The listing builds one solid part. Answer for the finished solid, in the listing's coordinates (mm). Face numbers are marked on the shaded views. A direction names the side the tool comes from. Coordinates: 2 decimals unless noted, no trailing zeros. Write each loop counter-clockwise with the first axis right and the second up, starting at its lowest first coordinate (ties: lowest second). Pieces come first, ordered by that corner, then holes.
```python
from build123d import *

# Parameters (mm, degrees)
SKETCH1_R                                    = 1.5
BOSS_EXTRUDE1_DEPTH                          = 1.2
BOSS_EXTRUDE1_2_DEPTH                        = 1.2
BOSS_EXTRUDE1_3_DEPTH                        = 1.2
SKETCH2_R                                    = 1.5
BOSS_EXTRUDE2_DEPTH                          = 3.5
SKETCH3_R                                    = 1.5
BOSS_EXTRUDE3_DEPTH                          = 1
CSK_FOR_M3_COUNTERSUNK_FLAT_HEAD_SCR_2_COUNT = 2
CSK_FOR_M3_COUNTERSUNK_FLAT_HEAD_SCR_2_PITCH = 19
CSK_FOR_M3_COUNTERSUNK_FLAT_HEAD_SCR_3_COUNT = 2
CSK_FOR_M3_COUNTERSUNK_FLAT_HEAD_SCR_3_PITCH = 38
SKETCH7_R                                    = 3
CUT_EXTRUDE1_DEPTH                           = 67.004185473
SKETCH8_W                                    = 6.5
SKETCH8_H                                    = 3.5
CUT_EXTRUDE2_DEPTH                           = 67.004185473
SKETCH10_W                                   = 9.5
SKETCH10_H                                   = 1.1
CUT_EXTRUDE3_DEPTH                           = 1


with BuildPart() as part:
    # Sketch1 → Boss-Extrude1 (new body)
    with BuildSketch(Plane.XY):
        Polygon((-55.55, 8.6), (-54.75, 8.6), (-54.75, 14), (-64.25, 14), (-64.25, 0), (-54.75, 0), (-54.75, 4.6), (-55.55, 4.6), align=None)
        with Locations((-59.5, 9.5)):
            Circle(SKETCH1_R, mode=Mode.SUBTRACT)
    extrude(amount=BOSS_EXTRUDE1_DEPTH)



with BuildPart() as body_2:
    # Sketch1 → Boss-Extrude1 2 (new body)
    with BuildSketch(Plane.XY):
        Polygon((-45.25, 4.6), (-45.25, 0), (-35.75, 0), (-35.75, 4.6), (-36.55, 4.6), (-36.55, 8.6), (-35.75, 8.6), (-35.75, 14), (-45.25, 14), (-45.25, 8.6), (-44.45, 8.6), (-44.45, 4.6), align=None)
        with Locations((-40.5, 9.5)):
            Circle(SKETCH1_R, mode=Mode.SUBTRACT)
    extrude(amount=BOSS_EXTRUDE1_2_DEPTH)


with BuildPart() as body_3:
    # Sketch1 → Boss-Extrude1 3 (new body)
    with BuildSketch(Plane.XY):
        Polygon((-26.25, 4.6), (-26.25, 0), (-16.75, 0), (-16.75, 14), (-26.25, 14), (-26.25, 8.6), (-25.45, 8.6), (-25.45, 4.6), align=None)
        with Locations((-21.5, 9.5)):
            Circle(SKETCH1_R, mode=Mode.SUBTRACT)
    extrude(amount=BOSS_EXTRUDE1_3_DEPTH)


with BuildPart() as part_1:
    add(part.part)

    add(body_2.part)  # Boss-Extrude2 merges body 2

    add(body_3.part)  # Boss-Extrude2 merges body 3
    # Sketch2 → Boss-Extrude2 (add)
    with BuildSketch(Plane.XY.offset(1.2)):
        Polygon((-54.75, 14), (-64.25, 14), (-64.25, 0), (-16.75, 0), (-16.75, 14), (-26.25, 14), (-26.25, 1.1), (-35.75, 1.1), (-35.75, 14), (-45.25, 14), (-45.25, 1.1), (-54.75, 1.1), align=None)
        with Locations((-59.5, 9.5)):
            Circle(SKETCH2_R, mode=Mode.SUBTRACT)
        with Locations((-40.5, 9.5)):
            Circle(SKETCH2_R, mode=Mode.SUBTRACT)
        with Locations((-21.5, 9.5)):
            Circle(SKETCH2_R, mode=Mode.SUBTRACT)
    extrude(amount=BOSS_EXTRUDE2_DEPTH)

    # Sketch3 → Boss-Extrude3 (add)
    with BuildSketch(Plane.XY.offset(4.7)):
        Polygon((-64.25, 14), (-54.75, 14), (-54.75, 12.1), (-45.25, 12.1), (-45.25, 14), (-35.75, 14), (-35.75, 12.1), (-26.25, 12.1), (-26.25, 14), (-16.75, 14), (-16.75, 0), (-64.25, 0), align=None)
        with Locations((-59.5, 9.5)):
            Circle(SKETCH3_R, mode=Mode.SUBTRACT)
        with Locations((-40.5, 9.5)):
            Circle(SKETCH3_R, mode=Mode.SUBTRACT)
        with Locations((-21.5, 9.5)):
            Circle(SKETCH3_R, mode=Mode.SUBTRACT)
    extrude(amount=BOSS_EXTRUDE3_DEPTH)

    # Sketch6 → CSK for M3 Countersunk Flat Head Screw1 (revolve, cut)
    with BuildSketch(Plane(origin=(-59.5, 9.5, 5.7), x_dir=(0, -1, 0), z_dir=(1, 0, 0))):
        Polygon((0, 0), (0, 5.7), (1.7, 5.7), (1.7, 1.75), (3.15, 0.3), (3.15, 0), align=None)
    csk_for_m3_countersunk_flat_head_screw1 = revolve(axis=Axis((-59.5, 9.5, 12.05), (0, 0, -1)), mode=Mode.SUBTRACT)

    # CSK for M3 Countersunk Flat Head Scr 2: CSK for M3 Countersunk Flat Head Screw1 ×2
    with Locations(*[(i * CSK_FOR_M3_COUNTERSUNK_FLAT_HEAD_SCR_2_PITCH, 0, 0) for i in range(1, CSK_FOR_M3_COUNTERSUNK_FLAT_HEAD_SCR_2_COUNT)]):
        add(csk_for_m3_countersunk_flat_head_screw1, mode=Mode.SUBTRACT)

    # CSK for M3 Countersunk Flat Head Scr 3: CSK for M3 Countersunk Flat Head Screw1 ×2
    with Locations(*[(i * CSK_FOR_M3_COUNTERSUNK_FLAT_HEAD_SCR_3_PITCH, 0, 0) for i in range(1, CSK_FOR_M3_COUNTERSUNK_FLAT_HEAD_SCR_3_COUNT)]):
        add(csk_for_m3_countersunk_flat_head_screw1, mode=Mode.SUBTRACT)

    # Sketch7 → Cut-Extrude1 (cut, through all)
    with BuildSketch(Plane.XY.offset(5.7)):
        with Locations((-50, 6)):
            Circle(SKETCH7_R)
        with Locations((-31, 6)):
            Circle(SKETCH7_R)
    extrude(amount=-CUT_EXTRUDE1_DEPTH, mode=Mode.SUBTRACT)

    # Sketch8 → Cut-Extrude2 (cut, through all)
    with BuildSketch(Plane.XY.offset(5.7)):
        with Locations((-61, 1.75)):
            Rectangle(SKETCH8_W, SKETCH8_H)
        with Locations((-20, 1.75)):
            Rectangle(SKETCH8_W, SKETCH8_H)
    extrude(amount=-CUT_EXTRUDE2_DEPTH, mode=Mode.SUBTRACT)

    # Sketch10 → Cut-Extrude3 (cut)
    with BuildSketch(Plane(origin=(0, 0, 1.2), x_dir=(-1, 0, 0), z_dir=(0, 0, -1))):
        with Locations((31, 0.55)):
            Rectangle(SKETCH10_W, SKETCH10_H)
        with Locations((50, 0.55)):
            Rectangle(SKETCH10_W, SKETCH10_H)
    extrude(amount=-CUT_EXTRUDE3_DEPTH, mode=Mode.SUBTRACT)


solid = part_1.part
```
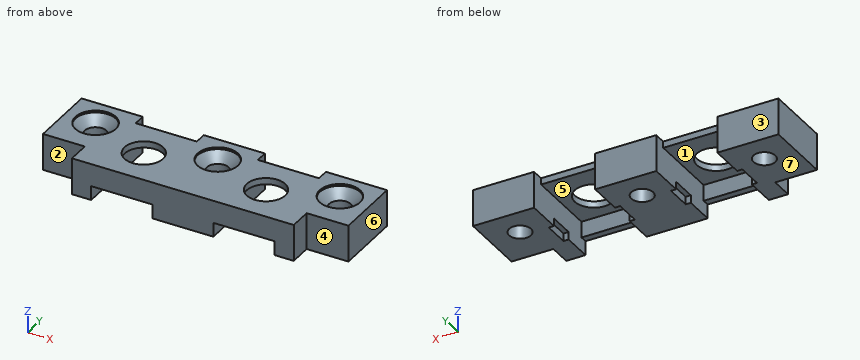
(1) Which of the six approach directions +Z, -Z, +X, -X, +Y, -Y give full straight-line access (tool end or side, diameter ignored) to the marked faces 1, 2, 3 and 4?
(2) Find the intervals of material crossed by probe 1 along X at (y, z) = (9.5, 5.6); probe 2 along X at (y, z) = (5.5, 2.85); probe 3 along Y at (x, z) = (-59.5, 5.5), in increasing order.
(3) Section D-D, the plane y = 9.5 is taken. State how many separate pieces and enclosed holes the cut face has, plus the area to 3 significant figures.
(4) Section A-A, the plane x = -50 is taken. Write down the section's boundary in (y, z), plus the area to 3 significant figures.
(5) For a pull along X with two mould halves and no side action, classify the marked faces 5, 6 and 7 as pulls with the +X half, pulls with the -X half, needs draft (parallel to the pull), parting line crosses it, or undercut.
(6) Each of these flat-tipped pins is pushed along its axis until it touches: pin 1 (3 mm diameter, centred on x = -18.5, z = 2.5, fed in from -Y); pin 2 (1.8 mm diameter, centred on y = 2, z = 2, fed in from -X); pin 3 (2 mm diameter, centred on x = -42.5, z = 1, fed in from -Y); pin 4 (0.5 mm diameter, centred on x = -49.5, z = 5, fed in from +Y). Where does it stop, or does it pass through?
(7) Section C-C, the plane y = 1.5 is taken. Write down the section's boundary in (x, z).
(8) Section B-B, the plane z = 3.55 is taken. Write down the section's boundary in (x, y).
Solution:
1. face 1: -Z, +Y
1. face 2: +Z, -Z, -X, -Y
1. face 3: +Z, -Z, +X, -X, +Y
1. face 4: +Z, -Z, +X, -Y
2. probe 1: x = -64.25 to -62.65, -56.35 to -43.65, -37.35 to -24.65, -18.35 to -16.75
2. probe 2: x = -64.25 to -54.75, -45.25 to -35.75, -26.25 to -16.75
2. probe 3: y = 3.5 to 6.35, 12.65 to 14
3. separate pieces: 4
3. enclosed holes: 0
3. area: 114 mm2
4. outline: (0, 2.2) - (1.1, 2.2) - (1.1, 4.7) - (3, 4.7) - (3, 5.7) - (0, 5.7) - close; (9, 4.7) - (12.1, 4.7) - (12.1, 5.7) - (9, 5.7) - close
4. area: 8.85 mm2
5. face 5: undercut
5. face 6: pulls with the +X half
5. face 7: needs draft
6. pin 1: stops at y = 3.5
6. pin 2: stops at x = -57.75
6. pin 3: stops at y = 0
6. pin 4: stops at y = 12.1
7. outline: (-57.75, 0) - (-54.75, 0) - (-54.75, 4.7) - (-45.25, 4.7) - (-45.25, 0) - (-35.75, 0) - (-35.75, 4.7) - (-26.25, 4.7) - (-26.25, 0) - (-23.25, 0) - (-23.25, 5.7) - (-57.75, 5.7) - close
8. outline: (-64.25, 3.5) - (-57.75, 3.5) - (-57.75, 0) - (-23.25, 0) - (-23.25, 3.5) - (-16.75, 3.5) - (-16.75, 14) - (-26.25, 14) - (-26.25, 1.1) - (-35.75, 1.1) - (-35.75, 14) - (-45.25, 14) - (-45.25, 1.1) - (-54.75, 1.1) - (-54.75, 14) - (-64.25, 14) - close; hole circle Ø3.4 at (-59.5, 9.5); hole circle Ø3.4 at (-40.5, 9.5); hole circle Ø3.4 at (-21.5, 9.5)
